```python
from build123d import *

# Parameters (mm, degrees)
SKETCH1_R           = 3.175
BOSS_EXTRUDE1_DEPTH = 50
CUT_EXTRUDE2_DEPTH  = 85
CUT_EXTRUDE3_DEPTH  = 5


with BuildPart() as part:
    # Sketch1 → Boss-Extrude1 (new, symmetric)
    with BuildSketch(Plane(origin=(0, 0, 0), x_dir=(0, 0, -1), z_dir=(1, 0, 0))):
        with BuildLine():
            Line((81.651944222, 112.683382271), (59.836598551, 46.569389334))
            Line((59.836598551, 46.569389334), (26.418811763, 131.99560075))
            ThreePointArc((26.418811763, 131.99560075), (17.598489936, 138.340405822), (8.196783623, 132.894072472))
            ThreePointArc((8.196783623, 132.894072472), (-6.288509671, 122.256846087), (-23.465130006, 127.542488985))
            ThreePointArc((-23.465130006, 127.542488985), (-41.174252563, 132.730696676), (-55.592419973, 121.213450072))
            Line((-55.592419973, 121.213450072), (-111.125559912, -4.052805204))
            ThreePointArc((-111.125559912, -4.052805204), (-124.320288873, -9.141923757), (-129.409407426, 4.052805204))
            Line((-129.409407426, 4.052805204), (-53.514907077, 175.248236709))
            Line((-53.514907077, 175.248236709), (10.663375069, 175.248236709))
            Line((10.663375069, 175.248236709), (81.651944222, 112.683382271))
        make_face()
        with Locations(Location((-120.267483669, 0, 0), (0, 0, 180))):
            Circle(SKETCH1_R, mode=Mode.SUBTRACT)
        with Locations(Location((-9.621687552, 141.977138307, 0), (0, 0, 180))):
            Circle(SKETCH1_R, mode=Mode.SUBTRACT)
    extrude(amount=BOSS_EXTRUDE1_DEPTH, both=True)

    # Sketch3 → Cut-Extrude2 (cut)
    with BuildSketch(Plane(origin=(0, -60.961450511, 158.231581065), x_dir=(1, 0, 0), z_dir=(0, -0.40528052042874013, -0.9141923756852326))):
        Polygon((50, -254.130320218), (10, -254.130320218), (10, -103.605584332), (4.413734497, -103.605584332), (4.413734497, -45.786353236), (50, -45.786353236), align=None)
        Polygon((-50, -254.130320218), (-50, -45.786353236), (-4.413734497, -45.786353236), (-4.413734497, -103.605584332), (-10, -103.605584332), (-10, -254.130320218), align=None)
    extrude(amount=CUT_EXTRUDE2_DEPTH, mode=Mode.SUBTRACT)

    # Sketch4 → Cut-Extrude3 (cut, symmetric)
    with BuildSketch(Plane(origin=(0, 0, 0), x_dir=(0, 0, -1), z_dir=(1, 0, 0))):
        Polygon((-15.368692055, 153.687872136), (12.057079216, 141.529456524), (-11.845454529, 87.612445941), (-39.271225799, 99.770861554), align=None)
    extrude(amount=CUT_EXTRUDE3_DEPTH, both=True, mode=Mode.SUBTRACT)


solid = part.part
```
Part model, mm, in its own coordinate system. A direction names the side the tool comes from. Round coordinates to 2 decimals unless told otherwise and drop trailing zeros. Write each loop counter-clockwise with the first axis right and the second up, starting at its lowest first coordinate (ties: lowest second). Pieces come first, ordered by that corner, then holes. Notation, with made-up numbers: (82, 0.25) -> (124, 0.25) arc R16 ccw to (124, 10.25) -> close; hole circle Ø1 at (37, -25). An arc over 180 degrees is marked (long way). Return JSON: item names as keys, results as strings. Group by question number.
Q1. Saw through at C-C on z = 107. Write the cut outline in (x, y).
Q2. Saw through at A-A on y = 97. Write the cut outline in (x, z).
Q3. Mould opens along Y. For faces 1 (the cylindrical face through (-7.535, 145.077, 8.933)), 2 (the flat face through (0.233, 108.273, 83.207)), 3 (the flat face through (-7.17, 29.76, 107.23)), 4 (the cylindrical face through (-0.062, -0.14, 117.096)) say: pulls with the +Y half, pulls with the -Y half, needs draft (parallel to the pull), parting line crosses it, or undercut.
Q4. Probe L1, parallel to Z at x = -3.5, y = 136; L2, parallel to X at y = 154, z = 56; L3, parallel to Z at x = -7.5, y = 103. List the from-to ranges inside material, lowest first. Write a range as [from, to].
Q5. Pin check, flat tips, straight feed: pin 1 (9.5 mm diameter, centred on y = 6, z = 118.5, fed in from +X); pin 2 (4 mm diameter, centred on y = 0, z = 120.27, fed in from -X); pin 3 (2 mm diameter, centred on x = 5, z = 108.5, fed in from +Y); pin 4 (10 mm diameter, centred on y = 141.98, z = 9.62, fed in from +X). Stop position of each tip, or through.
Q6. Which spindle directions (+Z, -Z, +X, -X, +Y, -Y) get a long thin tool onto all of the face, cutting with end or side? Do faces 5 (the flat face through (0.07, 141.489, 20.777)), 6 (the flat face through (0.14, 59.46, 82.97)), 7 (the flat face through (-29.72, 154.38, 16.93)), 8 (the flat face through (10, 113, 66)), 9 (the flat face through (1, 175.248, 22)). Say none if no direction does.
Q7. Saw through at D-D on y = 0. Write the cut outline in (x, z), plus the area to 3 significant figures.
Q8. Saw through at B-B on x = 33.5. Write the cut outline in (y, z), plus the area to 3 significant figures.
Answer:
{
 "1": {"outline": "(-10, 29.66) -> (-4.41, 29.66) -> (-4.41, 5.25) -> (4.41, 5.25) -> (4.41, 29.66) -> (10, 29.66) -> (10, 54.6) -> (-10, 54.6) -> close"},
 "2": {"outline": "(-50, -76.48) -> (50, -76.48) -> (50, -40.11) -> (-50, -40.11) -> close; (-10, 66.33) -> (10, 66.33) -> (10, 88.2) -> (-10, 88.2) -> close"},
 "3": {"face 1": "undercut", "face 2": "pulls with the +Y half", "face 3": "pulls with the -Y half", "face 4": "undercut"},
 "4": {"L1": "[-55.2, -23.55], [-10.66, -9.61], [23.21, 70.91]", "L2": "[-10, 10]", "L3": "[-78.46, -37.76], [63.67, 85.54]"},
 "5": {"pin 1": "x = 4.41", "pin 2": "through", "pin 3": "y = 53.47", "pin 4": "x = 10"},
 "6": {"face 5": "-Y", "face 6": "+X, -X, -Y", "face 7": "+Z, -X, -Y", "face 8": "+Z, +X, -Y", "face 9": "+Z, -Z, +X, -X, +Y"},
 "7": {"outline": "(-4.41, 109.33) -> (4.41, 109.33) -> (4.41, 117.09) -> (-4.41, 117.09) -> close; (-4.41, 123.44) -> (4.41, 123.44) -> (4.41, 130.27) -> (-4.41, 130.27) -> close", "area": "129 mm2"},
 "8": {"outline": "(46.57, -59.84) -> (112.68, -81.65) -> (175.25, -10.66) -> (175.25, 53.51) -> (171.36, 55.24) -> (136.91, -22.47) -> (136.82, -22.43) arc R10 cw to (132, -26.42) -> close", "area": "4,530 mm2"}
}
